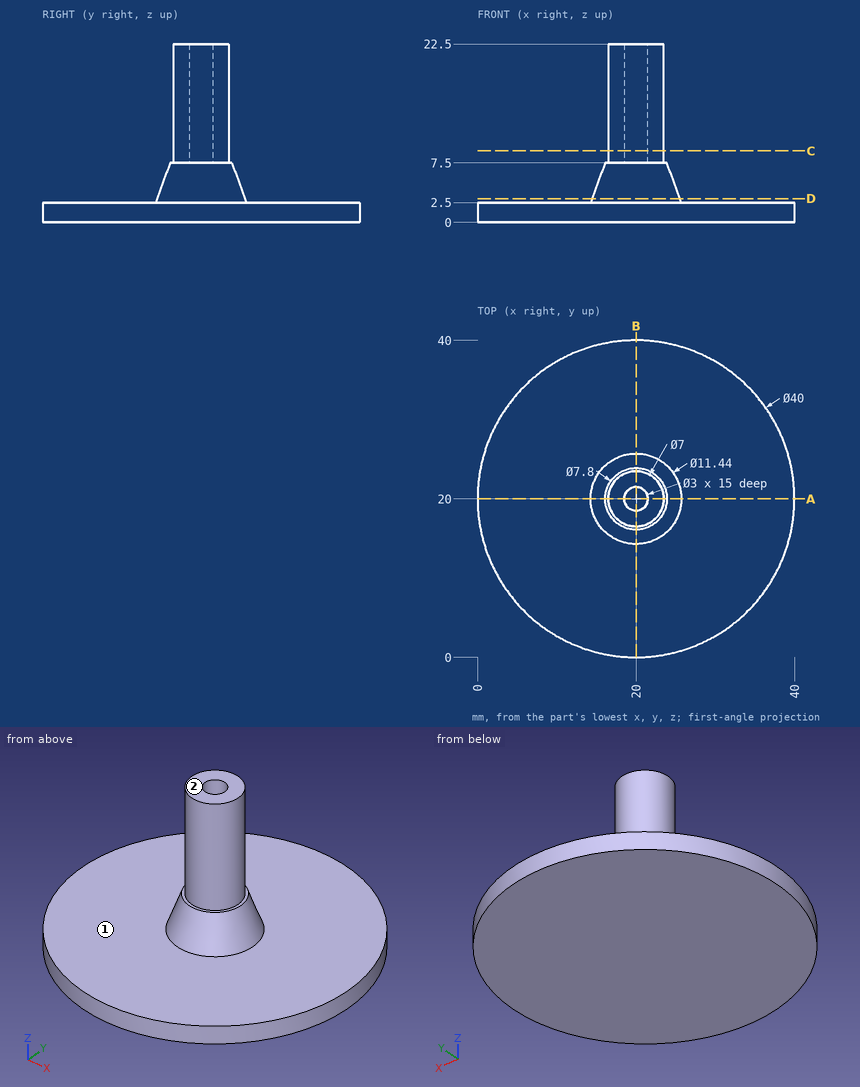
Can you work these out from the drawing? Everything is in mm from the part's minimum corner. A direction names the side the tool comes from. Give positions to 0.01 mm unless a question says otherwise; leave off trailing zeros. Order: outer loops, then holes, each group sorted by start corner. A loop starts at its lowest first (then second) coordinate and runs counter-clockwise, first axis right, second up.
1. Suppose I cut it at C-C (z = 9). List the corners of the cut face in (x, y) for me.
2. I need wall thicknesses on L1, parallel to X at y = 20, z = 17.25; L2, parallel to Z at x = 38, y = 16. Which ranges of each line are inside material? Lowest first, please.
3. Will these pins go through, and if not, where does the flat tip stop? P1, Ø4, axis at x = 24.5, z = 11.5, coming from the +Y side; P2, Ø5, axis at x = 19, z = 19.5, coming from the -Y side; P3, Ø12, axis at y = 11.5, z = 13, coming from the +X side.
4. Suppose I cut it at D-D (z = 3). List the corners of the cut face in (x, y) for me (1 decimal).
5. For the marked faces 1 and 2, which set-ups out of +Z, -Z, +X, -X, +Y, -Y let a thin tool reach every point of the face, with its end or its side?
6. Suppose I cut it at A-A (y = 20). List the corners of the cut face in (x, z) for me, plus the area to 3 significant figures.
Solved:
1. outline: circle Ø7 at (20, 20); hole circle Ø3 at (20, 20)
2. L1: x = 16.5 to 18.5, 21.5 to 23.5
2. L2: z = 0 to 2.5
3. P1: stops at y = 22.45
3. P2: stops at y = 16.5
3. P3: stops at x = 22.45
4. outline: circle Ø11.1 at (20, 20)
5. face 1: +Z
5. face 2: +Z, +X, -X, +Y, -Y
6. outline: (0, 0) - (40, 0) - (40, 2.5) - (25.72, 2.5) - (23.9, 7.5) - (23.5, 7.5) - (23.5, 22.5) - (21.5, 22.5) - (21.5, 7.5) - (18.5, 7.5) - (18.5, 22.5) - (16.5, 22.5) - (16.5, 7.5) - (16.1, 7.5) - (14.28, 2.5) - (0, 2.5) - close
6. area: 208 mm2
